Read the model definition and answer for the solid it produces. Units are mm, in the model's axes. A direction names the side the tool comes from. Coordinates: 2 decimals unless noted, no trailing zeros. Write each loop counter-clockwise with the first axis right and the second up, starting at its lowest first coordinate (ties: lowest second). Pieces come first, ordered by that corner, then holes. Notation, with made-up numbers: (20.5, 15) -> (54.5, 15) arc R18 ccw to (54.5, 23) -> close; hole circle Ø2 at (-18.5, 34). An arc over 180 degrees is marked (long way). One line per item, written item: value. Start each with the question number.
1. For faces 5 (the flat face through (-9, 0, 10)), 6 (the flat face through (-6.587, 18.662, 44.93)), determine the directions among +Z, -Z, +X, -X, +Y, -Y from which every point of the face is accessible in a straight line to the end or side of a thin tool.
2. Find section A-A, the plane y = 0. Write down the section's boundary in (x, z), and give its area (3 significant figures).
3. Find section C-C, the plane z = 42. Write down the section's boundary in (x, y).
4. Find section B-B, the plane x = 2. Write down the section's boundary in (y, z).
5. Given P1, Ø6, axis at x = 0.5, z = 5, coming from the -Y side; P2, Ø9, axis at y = 12.5, z = 27.5, coming from the +X side; P3, Ø1, axis at x = -12, z = 7.5, coming from the -Y side, each flat-ended and moving along its own axis, determine where each tip first touches the part or whether it passes through.
6. For a pull along X with two mould halves and no side action, classify faces 1 (the flat face through (-30, 0, 25)), 2 (the flat face through (-15, 0, 50)), 3 (the flat face through (-20, 0, 25)), 4 (the cylindrical face through (-0.867, -3.905, 4.93)) as pulls with the +X half, pulls with the -X half, needs draft (parallel to the pull), parting line crosses it, or undercut.
7. Consider line 1 along Z through (x, y) = (-4, 2); line 2 along X through (y, z) = (18, 12.5); line 3 along Y through (x, z) = (-3.5, 43.5). Determine where each line is inside the solid, lowest interval first.
8. Find section D-D, the plane x = -14. Write down the section's boundary in (y, z), and give its area (3 significant figures).
```python
from build123d import *

# Parameters (mm, degrees)
SKETCH1_R               = 4
BOSS_EXTRUDE1_DEPTH     = 50
CUT_EXTRUDE1_DEPTH      = 40
CUT_EXTRUDE1_DEPTH_BACK = 20
SKETCH2_W               = 30
SKETCH2_H               = 60


with BuildPart() as part:
    # Sketch1 → Boss-Extrude1 (new body)
    with BuildSketch(Plane.XY):
        with BuildLine():
            ThreePointArc((6.455619112, -7.637079408), (10, 0), (6.455619112, 7.637079408))
            Line((6.455619112, 7.637079408), (-20, 30))
            Line((-20, 30), (-30, 30))
            Line((-30, 30), (-30, -30))
            Line((-30, -30), (-20, -30))
            Line((-20, -30), (6.455619112, -7.637079408))
        make_face()
        Circle(SKETCH1_R, mode=Mode.SUBTRACT)
    extrude(amount=BOSS_EXTRUDE1_DEPTH)

    # Sketch2 → Cut-Extrude1 (cut, two sides: drawn at the far end of the back side and taken through both)
    with BuildSketch(Plane(origin=(0, 0, 0), x_dir=(0, 0, -1), z_dir=(1, 0, 0)).offset(-CUT_EXTRUDE1_DEPTH_BACK)):
        with Locations((-25, 0)):
            Rectangle(SKETCH2_W, SKETCH2_H)
    extrude(amount=CUT_EXTRUDE1_DEPTH + CUT_EXTRUDE1_DEPTH_BACK, mode=Mode.SUBTRACT)


solid = part.part
```
Answer block:
1. face 5: +X, +Y, -Y
1. face 6: +Z, -Z, +X, +Y
2. outline: (-30, 0) -> (-4, 0) -> (-4, 10) -> (-20, 10) -> (-20, 40) -> (-4, 40) -> (-4, 50) -> (-30, 50) -> close; (4, 0) -> (10, 0) -> (10, 10) -> (4, 10) -> close; (4, 40) -> (10, 40) -> (10, 50) -> (4, 50) -> close
2. area: 940 mm2
3. outline: (-30, -30) -> (-20, -30) -> (6.46, -7.64) arc R10 ccw to (6.46, 7.64) -> (-20, 30) -> (-30, 30) -> close; hole circle Ø8 at (0, 0)
4. outline: (-11.4, 0) -> (-3.46, 0) -> (-3.46, 10) -> (-11.4, 10) -> close; (-11.4, 40) -> (-3.46, 40) -> (-3.46, 50) -> (-11.4, 50) -> close; (3.46, 0) -> (11.4, 0) -> (11.4, 10) -> (3.46, 10) -> close; (3.46, 40) -> (11.4, 40) -> (11.4, 50) -> (3.46, 50) -> close
5. P1: stops at y = -15.21
5. P2: stops at x = -20
5. P3: stops at y = -23.66
6. face 1: pulls with the -X half
6. face 2: needs draft
6. face 3: pulls with the +X half
6. face 4: undercut
7. line 1: z = 0 to 10, 40 to 50
7. line 2: x = -30 to -20
7. line 3: y = -16.05 to -1.94, 1.94 to 16.05
8. outline: (-24.93, 0) -> (24.93, 0) -> (24.93, 10) -> (-24.93, 10) -> close; (-24.93, 40) -> (24.93, 40) -> (24.93, 50) -> (-24.93, 50) -> close
8. area: 997 mm2
